```python
from build123d import *

# Parameters (mm, degrees)
F0_W      = 15
F0_H      = 15
F1_DEPTH  = 15
F2_R      = 2
F3_DEPTH  = 1
F4_R      = 1.5
F5_DEPTH  = 1
F6_R      = 1.5
F7_DEPTH  = 1
F8_R      = 1.5
F9_DEPTH  = 1
F10_R     = 1.5
F11_DEPTH = 1
F12_R     = 1.5
F13_DEPTH = 1
F15_SIZE  = 0.2


# Not quite as in the source:
# - a fillet or chamfer that OpenCascade refuses, or shapes differently, is made with other operations: its cross-section is extruded or revolved along the edge and cut away or added


with BuildPart() as f1:
    # F0 (on Top) → F1 (new body)
    with BuildSketch(Plane.XY):
        with Locations((7.5, 7.5)):
            Rectangle(F0_W, F0_H)
    extrude(amount=F1_DEPTH)

    # F2 (on face) → F3 (cut)
    with BuildSketch(Plane.XY.offset(15)):
        with Locations((7.5, 7.5)):
            Circle(F2_R)
    extrude(amount=-F3_DEPTH, mode=Mode.SUBTRACT)

    # F4 (on face) → F5 (cut)
    with BuildSketch(Plane(origin=(0, 0, 0), x_dir=(1, 0, 0), z_dir=(0, 0, -1))):
        with Locations((5, -3.75)):
            Circle(F4_R)
        with Locations((10, -3.75)):
            Circle(F4_R)
        with Locations((10, -7.5)):
            Circle(F4_R)
        with Locations((5, -7.5)):
            Circle(F4_R)
        with Locations((5, -11.25)):
            Circle(F4_R)
        with Locations((10, -11.25)):
            Circle(F4_R)
    extrude(amount=-F5_DEPTH, mode=Mode.SUBTRACT)

    # F6 (on face) → F7 (cut)
    with BuildSketch(Plane.YZ.offset(15)):
        with Locations((3.75, 3.75)):
            Circle(F6_R)
        with Locations((11.25, 11.25)):
            Circle(F6_R)
    extrude(amount=-F7_DEPTH, mode=Mode.SUBTRACT)

    # F8 (on face) → F9 (cut)
    with BuildSketch(Plane(origin=(0, 0, 0), x_dir=(0, -1, 0), z_dir=(-1, 0, 0))):
        with Locations((-11.25, 11.25)):
            Circle(F8_R)
        with Locations((-7.5, 7.5)):
            Circle(F8_R)
        with Locations((-11.25, 3.75)):
            Circle(F8_R)
        with Locations((-3.75, 3.75)):
            Circle(F8_R)
        with Locations((-3.75, 11.25)):
            Circle(F8_R)
    extrude(amount=-F9_DEPTH, mode=Mode.SUBTRACT)

    # F10 (on face) → F11 (cut)
    with BuildSketch(Plane(origin=(0, 15, 0), x_dir=(-1, 0, 0), z_dir=(0, 1, 0))):
        with Locations((-3.75, 11.25)):
            Circle(F10_R)
        with Locations((-7.5, 7.5)):
            Circle(F10_R)
        with Locations((-11.25, 3.75)):
            Circle(F10_R)
    extrude(amount=-F11_DEPTH, mode=Mode.SUBTRACT)

    # F12 (on face) → F13 (cut)
    with BuildSketch(Plane.XZ):
        with Locations((3.75, 11.25)):
            Circle(F12_R)
        with Locations((11.25, 11.25)):
            Circle(F12_R)
        with Locations((11.25, 3.75)):
            Circle(F12_R)
        with Locations((3.75, 3.75)):
            Circle(F12_R)
    extrude(amount=-F13_DEPTH, mode=Mode.SUBTRACT)

    # F14: fillet of radius 1.6 on 21 edges, made by hand

    # F14_s1 → F14_t2 (revolve)
    with BuildSketch(Plane.XY.offset(3.75)):
        with BuildLine():
            ThreePointArc((0, 9.75), (0.7266499161, 10.3388125064), (1, 11.2332396974))
            Line((1, 11.2332396974), (1, 9.75))
            Line((1, 9.75), (0, 9.75))
        make_face()
    revolve(axis=Axis((1, 11.25, 3.75), (-1, 0, 0)))

    # F14_s3 → F14_t4 (revolve)
    with BuildSketch(Plane.XY.offset(7.5)):
        with BuildLine():
            ThreePointArc((0, 6), (0.7266499161, 6.5888125064), (1, 7.4832396974))
            Line((1, 7.4832396974), (1, 6))
            Line((1, 6), (0, 6))
        make_face()
    revolve(axis=Axis((1, 7.5, 7.5), (-1, 0, 0)))

    # F14_s5 → F14_t6 (revolve)
    with BuildSketch(Plane.XY.offset(11.25)):
        with BuildLine():
            ThreePointArc((0, 9.75), (0.7266499161, 10.3388125064), (1, 11.2332396974))
            Line((1, 11.2332396974), (1, 9.75))
            Line((1, 9.75), (0, 9.75))
        make_face()
    revolve(axis=Axis((1, 11.25, 11.25), (-1, 0, 0)))

    # F14_s7 → F14_t8 (revolve)
    with BuildSketch(Plane.XY.offset(3.75)):
        with BuildLine():
            ThreePointArc((0, 2.25), (0.7266499161, 2.8388125064), (1, 3.7332396974))
            Line((1, 3.7332396974), (1, 2.25))
            Line((1, 2.25), (0, 2.25))
        make_face()
    revolve(axis=Axis((1, 3.75, 3.75), (-1, 0, 0)))

    # F14_s9 → F14_t10 (revolve)
    with BuildSketch(Plane.XY.offset(11.25)):
        with BuildLine():
            ThreePointArc((0, 2.25), (0.7266499161, 2.8388125064), (1, 3.7332396974))
            Line((1, 3.7332396974), (1, 2.25))
            Line((1, 2.25), (0, 2.25))
        make_face()
    revolve(axis=Axis((1, 3.75, 11.25), (-1, 0, 0)))

    # F14_s11 → F14_t12 (revolve)
    with BuildSketch(Plane.XY.offset(11.25)):
        with BuildLine():
            ThreePointArc((2.25, 15), (2.8388125064, 14.2733500839), (3.7332396974, 14))
            Line((3.7332396974, 14), (2.25, 14))
            Line((2.25, 14), (2.25, 15))
        make_face()
    revolve(axis=Axis((3.75, 14, 11.25), (0, 1, 0)))

    # F14_s13 → F14_t14 (revolve)
    with BuildSketch(Plane.XY.offset(7.5)):
        with BuildLine():
            ThreePointArc((6, 15), (6.5888125064, 14.2733500839), (7.4832396974, 14))
            Line((7.4832396974, 14), (6, 14))
            Line((6, 14), (6, 15))
        make_face()
    revolve(axis=Axis((7.5, 14, 7.5), (0, 1, 0)))

    # F14_s15 → F14_t16 (revolve)
    with BuildSketch(Plane.XY.offset(3.75)):
        with BuildLine():
            ThreePointArc((9.75, 15), (10.3388125064, 14.2733500839), (11.2332396974, 14))
            Line((11.2332396974, 14), (9.75, 14))
            Line((9.75, 14), (9.75, 15))
        make_face()
    revolve(axis=Axis((11.25, 14, 3.75), (0, 1, 0)))

    # F14_s17 → F14_t18 (revolve)
    with BuildSketch(Plane.XZ.offset(-11.25)):
        with BuildLine():
            ThreePointArc((11.5, 0), (10.9111874936, 0.7266499161), (10.0167603026, 1))
            Line((10.0167603026, 1), (11.5, 1))
            Line((11.5, 1), (11.5, 0))
        make_face()
    revolve(axis=Axis((10, 11.25, 1), (0, 0, -1)))

    # F14_s19 → F14_t20 (revolve)
    with BuildSketch(Plane.XZ.offset(-7.5)):
        with BuildLine():
            ThreePointArc((11.5, 0), (10.9111874936, 0.7266499161), (10.0167603026, 1))
            Line((10.0167603026, 1), (11.5, 1))
            Line((11.5, 1), (11.5, 0))
        make_face()
    revolve(axis=Axis((10, 7.5, 1), (0, 0, -1)))

    # F14_s21 → F14_t22 (revolve)
    with BuildSketch(Plane.XZ.offset(-11.25)):
        with BuildLine():
            ThreePointArc((6.5, 0), (5.9111874936, 0.7266499161), (5.0167603026, 1))
            Line((5.0167603026, 1), (6.5, 1))
            Line((6.5, 1), (6.5, 0))
        make_face()
    revolve(axis=Axis((5, 11.25, 1), (0, 0, -1)))

    # F14_s23 → F14_t24 (revolve)
    with BuildSketch(Plane.XZ.offset(-7.5)):
        with BuildLine():
            ThreePointArc((6.5, 0), (5.9111874936, 0.7266499161), (5.0167603026, 1))
            Line((5.0167603026, 1), (6.5, 1))
            Line((6.5, 1), (6.5, 0))
        make_face()
    revolve(axis=Axis((5, 7.5, 1), (0, 0, -1)))

    # F14_s25 → F14_t26 (revolve)
    with BuildSketch(Plane.XZ.offset(-3.75)):
        with BuildLine():
            ThreePointArc((6.5, 0), (5.9111874936, 0.7266499161), (5.0167603026, 1))
            Line((5.0167603026, 1), (6.5, 1))
            Line((6.5, 1), (6.5, 0))
        make_face()
    revolve(axis=Axis((5, 3.75, 1), (0, 0, -1)))

    # F14_s27 → F14_t28 (revolve)
    with BuildSketch(Plane.XZ.offset(-3.75)):
        with BuildLine():
            ThreePointArc((11.5, 0), (10.9111874936, 0.7266499161), (10.0167603026, 1))
            Line((10.0167603026, 1), (11.5, 1))
            Line((11.5, 1), (11.5, 0))
        make_face()
    revolve(axis=Axis((10, 3.75, 1), (0, 0, -1)))

    # F14_s29 → F14_t30 (revolve)
    with BuildSketch(Plane.XY.offset(3.75)):
        with BuildLine():
            ThreePointArc((15, 5.25), (14.2733500839, 4.6611874936), (14, 3.7667603026))
            Line((14, 3.7667603026), (14, 5.25))
            Line((14, 5.25), (15, 5.25))
        make_face()
    revolve(axis=Axis((14, 3.75, 3.75), (1, 0, 0)))

    # F14_s31 → F14_t32 (revolve)
    with BuildSketch(Plane.XY.offset(11.25)):
        with BuildLine():
            ThreePointArc((15, 12.75), (14.2733500839, 12.1611874936), (14, 11.2667603026))
            Line((14, 11.2667603026), (14, 12.75))
            Line((14, 12.75), (15, 12.75))
        make_face()
    revolve(axis=Axis((14, 11.25, 11.25), (1, 0, 0)))

    # F14_s33 → F14_t34 (revolve)
    with BuildSketch(Plane.XZ.offset(-7.5)):
        with BuildLine():
            ThreePointArc((9.5, 15), (8.9111874936, 14.2733500839), (8.0167603026, 14))
            Line((8.0167603026, 14), (9.5, 14))
            Line((9.5, 14), (9.5, 15))
        make_face()
    revolve(axis=Axis((7.5, 7.5, 14), (0, 0, 1)))

    # F14_s35 → F14_t36 (revolve)
    with BuildSketch(Plane.XY.offset(11.25)):
        with BuildLine():
            ThreePointArc((5.25, 0), (4.6611874936, 0.7266499161), (3.7667603026, 1))
            Line((3.7667603026, 1), (5.25, 1))
            Line((5.25, 1), (5.25, 0))
        make_face()
    revolve(axis=Axis((3.75, 1, 11.25), (0, -1, 0)))

    # F14_s37 → F14_t38 (revolve)
    with BuildSketch(Plane.XY.offset(11.25)):
        with BuildLine():
            ThreePointArc((12.75, 0), (12.1611874936, 0.7266499161), (11.2667603026, 1))
            Line((11.2667603026, 1), (12.75, 1))
            Line((12.75, 1), (12.75, 0))
        make_face()
    revolve(axis=Axis((11.25, 1, 11.25), (0, -1, 0)))

    # F14_s39 → F14_t40 (revolve)
    with BuildSketch(Plane.XY.offset(3.75)):
        with BuildLine():
            ThreePointArc((12.75, 0), (12.1611874936, 0.7266499161), (11.2667603026, 1))
            Line((11.2667603026, 1), (12.75, 1))
            Line((12.75, 1), (12.75, 0))
        make_face()
    revolve(axis=Axis((11.25, 1, 3.75), (0, -1, 0)))

    # F14_s41 → F14_t42 (revolve)
    with BuildSketch(Plane.XY.offset(3.75)):
        with BuildLine():
            ThreePointArc((5.25, 0), (4.6611874936, 0.7266499161), (3.7667603026, 1))
            Line((3.7667603026, 1), (5.25, 1))
            Line((5.25, 1), (5.25, 0))
        make_face()
    revolve(axis=Axis((3.75, 1, 3.75), (0, -1, 0)))

    # F15
    f15_edges = [f1.edges().sort_by_distance(p)[0] for p in [
        (15, 0, 7.5),
        (7.5, 0, 0),
        (15, 7.5, 0),
        (0, 7.5, 0),
        (0, 0, 7.5),
        (0, 15, 7.5),
        (7.5, 15, 0),
        (7.5, 15, 15),
        (0, 7.5, 15),
        (7.5, 0, 15),
        (15, 7.5, 15),
        (15, 15, 7.5),
    ]]
    chamfer(f15_edges, length=F15_SIZE)


solid = f1.part
```
Verification items for the finished model (mm, model axes). Coordinates: 2 decimals unless noted, no trailing zeros. Answer as a JSON object with one key per item and string values. Group by question number.
(1) Gauge pin test, flat end, axial feed: pin 1 (0.5 mm diameter, centred on x = 7.5, y = 7.5, fed in from +Z). Record the tip position at first contact, or that the pin passes through.
(2) Material ranges on line 1 (Z direction, x = 11, y = 7.75); line 2 (Z direction, x = 6.25, y = 8.75); line 3 (X direction, y = 6.25, z = 7.25), recorded low to high.
(3) Release check for a two-part mould opening along X. For faces 1 (the face through (9, 9.2, 15)), 2 (the face through (0, 7.4, 5.8)), 3 (the face through (7.5, 7.5, 14)) record: +X half, -X half, draft (parallel to the pull), parting line (faces both ways), or undercut.
Reply:
{
 "1": {"pin 1": "z = 14"},
 "2": {"line 1": "0.64 to 15", "line 2": "0 to 14.6", "line 3": "0.39 to 15"},
 "3": {"face 1": "draft", "face 2": "-X half", "face 3": "undercut"}
}
